The model under review builds one solid part; all positions refer to its coordinate system, in mm. A direction names the side the tool comes from. Give positions to 0.01 mm unless a question says otherwise; leave off trailing zeros. Loops run counter-clockwise (first coordinate to the right, second up) from the corner with the lowest first, then second, coordinate; pieces in that order, holes last. Notation, with made-up numbers: (62.5, 25) -> (80.5, 25) arc R30 cw to (80.5, 49) -> close; hole circle Ø1 at (42, 29). An arc over 180 degrees is marked (long way). Write each question's results on one line, items separated by ' | '. Start each with the question number.
Q1. Machinability: for faces 1 (the face through (-3.47, 15.62, 40.71)), 2 (the face through (-3.068, -17.827, 6.651)), which of the approach directions +Z, -Z, +X, -X, +Y, -Y give a long, thin tool a straight path to every point of the face, cutting with its end or side? Answer none if there is none.
Q2. Wall thickness on L1, parallel to Z at x = 15, y = 20.5; L2, parallel to Z at x = -13, y = -18.5; L3, parallel to Y at x = 10, z = 6.5: over which ranges is each line inside the solid? List them lowest first. Write a range as [from, to].
Q3. We need section A-A (y = 0). Write out the cut boundary in (x, z), plus the area to 3 significant figures.
Q4. Mouldability with a two-part tool opening along Y and no side actions: class faces 3 (the face through (-3.068, 17.828, 6.491)), 4 (the face through (6.691, 12.864, 30.566)), 5 (the face through (-3, 24, 10)), 6 (the face through (-13, 11, 20)) as released by +Y, released by -Y, zero draft, split by the parting line, or undercut.
Q5. Insertion check: pin 1 Ø1.9 at (y, z) = (19.44, 6.28) entering from -X (3 decimals); pin 2 Ø12 at (x, z) = (-19.5, 52.5) entering from +Y; pin 3 Ø1.5 at (x, y) = (-13.5, 15) entering from +Z; pin 4 Ø2 at (y, z) = (-8, 52.5) entering from -X. Each pin has a flat end and moves straight along its axis. Give the tip position at first contact, or say it passes through.
Q6. We need section C-C (z = 37). Write out the cut boundary in (x, y), plus the area to 3 significant figures.
Q7. We need section B-B (x = -5). Write out the cut boundary in (y, z) (3 decimals), plus the area to 3 significant figures.
Q8. We need section D-D (x = 6.5). Write out the cut boundary in (y, z) (3 decimals).
Autodesk Fusion 360 part; units mm, degrees
sketch "Boceto8" plane through (0, 0, 0) normal (0, 0, 1) x (1, 0, 0)
sketch "Boceto9" plane through (0, 0, 0) normal (0, 0, 1) x (1, 0, 0)
  circle A0 centre (0, 0) radius 14.5
  line L0 (20, 0) -> (20, 20)
  line L1 (20, 0) -> (20, -20)
  circle A1 centre (0, 0) radius 16
  line L2 (20, 20) -> (20, 24)
  line L3 (20, -20) -> (20, -24)
  line L4 (20, -20) -> (20, -24)
  line L5 (20, 0) -> (20, 20)
  line L6 (20, 0) -> (20, -20)
  circle A2 centre (0, 0) radius 16
  circle A3 centre (0, 0) radius 14.5
  line L7 (20, 20) -> (20, 24)
  line L8 (-25.5, 24) -> (-25.5, -24)
  line L9 (-25.5, 24) -> (20, 24)
  line L10 (20, -24) -> (-25.5, -24)
  dimension "d26" = 29
  dimension "d27" = 20
  dimension "d36" = 32
  dimension "d63" = 29
  dimension "d64" = 20
  dimension "d65" = 32
extrude "Extruir8" add sketch "Boceto9" along normal blind 62 contours A1 A2
extrude "Extruir10" add sketch "Boceto9" along normal blind 20 contours L0 L1 L2 L3 L4 L5 L6 L7 L8 L9 L10
fillet "Empalme3" radius 3 4 edges at (-25.5, -24, 10) (-25.5, 24, 10) (20, 24, 10) (20, -24, 10)
hole "Agujero6" at (20, 19.4786, 14.6367) direction (-1, 0, 0) diameter 3.25 depth 80 tip angle 118
hole "Agujero7" at (20, 19.4389, 6.2793) direction (-1, 0, 0) diameter 3.25 depth 80 tip angle 118
sketch "Boceto11" plane through (20, 0, 0) normal (1, 0, 0) x (0, 1, 0)
  arc A0 (21, 6.7303) -> (21, 5.8282) centre (19.4389, 6.2793) ccw
  line L0 (21, 6.7303) -> (21, 14.0658)
  arc A1 (21, 15.2076) -> (21, 14.0658) centre (19.4786, 14.6367) ccw
  line L1 (21, 15.2076) -> (21, 20)
  line L2 (21, 20) -> (-21, 20)
  line L3 (-21, 20) -> (-21, 0)
  line L4 (-21, 0) -> (21, 0)
  line L5 (21, 0) -> (21, 5.8282)
hole "Agujero8" at (20, -19.3772, 14.6266) direction (-1, 0, 0) diameter 3.25 depth 80 tip angle 118
hole "Agujero9" at (20, -19.413, 6.2987) direction (-1, 0, 0) diameter 3.25 depth 80 tip angle 118
extrude "Extruir9" [suppressed]
Output:
1) face 1: +Z | face 2: +X, -X
2) L1: [0, 5.05], [7.51, 13.37], [15.9, 20] | L2: [0, 4.95], [7.64, 13.26], [15.99, 20] | L3: [-24, -21.03], [-17.8, -10.5], [10.5, 17.83], [21.05, 24]
3) outline: (-25.5, 0) -> (-14.5, 0) -> (-14.5, 62) -> (-16, 62) -> (-16, 20) -> (-25.5, 20) -> close; (14.5, 0) -> (20, 0) -> (20, 20) -> (16, 20) -> (16, 62) -> (14.5, 62) -> close | area: 456 mm2
4) face 3: undercut | face 4: undercut | face 5: released by +Y | face 6: zero draft
5) pin 1: through | pin 2: y = 8.59 | pin 3: z = 20 | pin 4: x = -14.39
6) outline: circle Ø32 at (0, 0); hole circle Ø29 at (0, 0) | area: 144 mm2
7) outline: (-24, 0) -> (-13.611, 0) -> (-13.611, 62) -> (-15.199, 62) -> (-15.199, 20) -> (-24, 20) -> close; (13.611, 0) -> (24, 0) -> (24, 20) -> (15.199, 20) -> (15.199, 62) -> (13.611, 62) -> close; hole circle Ø3.25 at (-19.413, 6.299); hole circle Ø3.25 at (-19.377, 14.627); hole circle Ø3.25 at (19.439, 6.279); hole circle Ø3.25 at (19.479, 14.637) | area: 516 mm2
8) outline: (-24, 0) -> (-12.961, 0) -> (-12.961, 62) -> (-14.62, 62) -> (-14.62, 20) -> (-24, 20) -> close; (12.961, 0) -> (24, 0) -> (24, 20) -> (14.62, 20) -> (14.62, 62) -> (12.961, 62) -> close; hole circle Ø3.25 at (-19.413, 6.299); hole circle Ø3.25 at (-19.377, 14.627); hole circle Ø3.25 at (19.439, 6.279); hole circle Ø3.25 at (19.479, 14.637)
